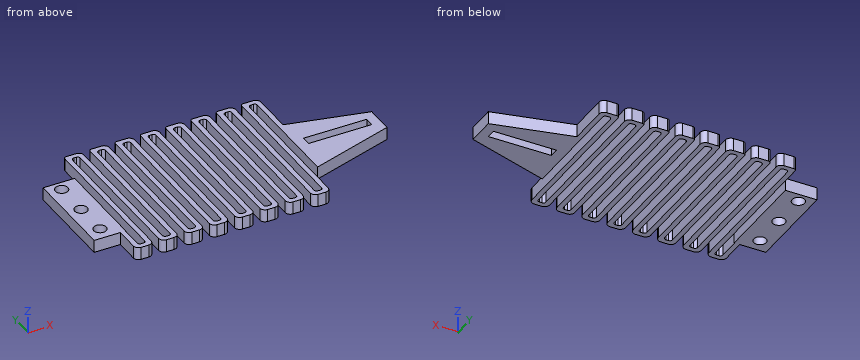
from build123d import *

# Parameters (mm, degrees)
F0_W      = 1.2
F0_H      = 0.8
F1_DEPTH  = 2
F2_R      = 0.4
F3_R      = 0.8
F11_DEPTH = 2
F14_DEPTH = 2
F15_R     = 1
F16_DEPTH = 2.001
F17_W     = 10
F17_H     = 1.5
F18_DEPTH = 2.001


with BuildPart() as f1:
    # F0 (on Top) → F1 (new body)
    with BuildSketch(Plane.XY):
        Polygon((8.5839435473, 25.4264183629), (8.5839435473, 13.2264183629), (9.3839435473, 13.2264183629), (9.3839435473, 26.2264183629), (6.5839435473, 26.2264183629), (6.5839435473, 2.0264183629), (6.5839435473, 1.2264183629), (7.3839435473, 1.2264183629), (7.3839435473, 25.4264183629), align=None)
        Polygon((4.5839435473, 1.2264183629), (5.3839435473, 1.2264183629), (5.3839435473, 2.0264183629), (5.3839435473, 14.2264183629), (4.5839435473, 14.2264183629), align=None)
        with Locations((5.9839435473, 1.6264183629)):
            Rectangle(F0_W, F0_H)
    extrude(amount=F1_DEPTH)

    # F2
    f2_edges = [f1.edges().sort_by_distance(p)[0] for p in [
        (7.383944, 25.426418, 1),
        (8.583944, 25.426418, 1),
        (5.383944, 2.026418, 1),
        (6.583944, 2.026418, 1),
        (6.583944, 26.226418, 1),
    ]]
    fillet(f2_edges, radius=F2_R)

    # F3
    f3_edges = [f1.edges().sort_by_distance(p)[0] for p in [
        (9.383944, 26.226418, 1),
        (7.383944, 1.226418, 1),
        (4.583944, 1.226418, 1),
    ]]
    fillet(f3_edges, radius=F3_R)


with BuildPart() as f4_1:
    # F4: copy of F1
    add(f1.part.moved(Location((4, 0, 0))))


with BuildPart() as f1_1:
    add(f1.part)

    # F5: union F4_1
    add(f4_1.part)


with BuildPart() as f6_1:
    # F6: copy of F1
    add(f1_1.part.moved(Location((8, 0, 0))))


with BuildPart() as f1_2:
    add(f1_1.part)

    # F7: union F6_1
    add(f6_1.part)


with BuildPart() as f8_1:
    # F8: copy of F1
    add(f1_2.part.moved(Location((16, 0, 0))))


with BuildPart() as f1_3:
    add(f1_2.part)

    # F9: union F8_1
    add(f8_1.part)

    # F10 (on face) → F11 (join)
    with BuildSketch(Plane.XY.offset(2)):
        Polygon((5.4478760238, 5.8683240786), (5.4478760238, 20.8683240786), (0.4478760238, 20.8683240786), (0.4478760238, 5.8683240786), (4.5839435473, 5.8683240786), (4.5839435473, 14.2264183629), (5.3839435473, 14.2264183629), (5.3839435473, 5.8683240786), align=None)
    extrude(amount=-F11_DEPTH)

    # F12: union 

    # F13 (on face) → F14 (join)
    with BuildSketch(Plane.XY.offset(2)):
        Polygon((49.8028248549, 15.969062224), (37.3839435473, 18.9353367689), (37.3839435473, 13.2264183629), (36.5839435473, 13.2264183629), (36.5839435473, 7.3133227415), (49.8028248549, 11.4841348702), align=None)
    extrude(amount=-F14_DEPTH)

    # F15 (on face) → F16 (cut, through all)
    with BuildSketch(Plane.XY.offset(2)):
        with Locations((2.5405562483, 19.2878898233)):
            Circle(F15_R)
        with Locations((2.5405562483, 13.5867726058)):
            Circle(F15_R)
        with Locations((2.5405562483, 8.0455001444)):
            Circle(F15_R)
    extrude(amount=-F16_DEPTH, mode=Mode.SUBTRACT)

    # F17 (on face) → F18 (cut, through all)
    with BuildSketch(Plane.XY.offset(2)):
        with Locations((43.2889471948, 13.8618260324)):
            Rectangle(F17_W, F17_H)
    extrude(amount=-F18_DEPTH, mode=Mode.SUBTRACT)


solid = f1_3.part
The listing builds one solid part. Answer for the finished solid, in the listing's coordinates (mm). Give positions to 0.01 mm unless a question says otherwise; leave off trailing zeros. Loops run counter-clockwise (first coordinate to the right, second up) from the corner with the lowest first, then second, coordinate; pieces in that order, holes last.
Item 1: A cutting plane is placed at A-A (x = 46). Give the vertices of the cut face in (y, z).
Derived:
outline: (10.28, 0) - (13.11, 0) - (13.11, 2) - (10.28, 2) - close; (14.61, 0) - (16.88, 0) - (16.88, 2) - (14.61, 2) - close
Item 2: A cutting plane is placed at B-B (y = 12). Give the number of separate pieces and of enclosed holes in the cut face, then the cut area to 3 significant figures.
Derived:
separate pieces: 17
enclosed holes: 0
area: 60.4 mm2
Item 3: Find the intervals of material crossed by line 1 along Y through (x, z) = (6, 1.9); line 2 along Y through (x, z) = (45, 1.05); line 3 along Y through (x, z) = (42, 1.7), in increasing order.
Derived:
line 1: y = 1.23 to 2.03
line 2: y = 9.97 to 13.11, 14.61 to 17.12
line 3: y = 9.02 to 13.11, 14.61 to 17.83
